```python
from build123d import *

# Parameters (mm, degrees)
SKETCH_W     = 130
SKETCH_H     = 110
PAD_DEPTH    = 1.6
SKETCH001_R  = 1.6
POCKET_DEPTH = 5


with BuildPart() as part:
    # Sketch → Pad (new body)
    with BuildSketch(Plane.XY):
        with Locations((65, 55)):
            Rectangle(SKETCH_W, SKETCH_H)
    extrude(amount=PAD_DEPTH)

    # Sketch001 → Pocket (cut)
    with BuildSketch(Plane.XY):
        with Locations((20, 20)):
            Circle(SKETCH001_R)
        with Locations((110, 89)):
            Circle(SKETCH001_R)
        with Locations((20, 90)):
            Circle(SKETCH001_R)
        with Locations((110, 20)):
            Circle(SKETCH001_R)
    extrude(amount=POCKET_DEPTH, mode=Mode.SUBTRACT)


solid = part.part
```
The listing builds one solid part. Answer for the finished solid, in the listing's coordinates (mm). Coordinates: 2 decimals unless noted, no trailing zeros. Write each loop counter-clockwise with the first axis right and the second up, starting at its lowest first coordinate (ties: lowest second). Pieces come first, ordered by that corner, then holes. Notation, with made-up numbers: (-37, 59) - (11, 59) arc R34 ccw to (11, 96) - close; hole circle Ø2 at (15, 15). An arc over 180 degrees is marked (long way). Return JSON: item names as keys, results as strings. Group by question number.
1. Determine the mould class of faces 1 (the cylindrical face through (19.792, 91.586, 0.789)), 2 (the flat face through (64, 56, 0)) for opening direction X: released by +X, released by -X, zero draft, split by the parting line, or undercut.
2. A cutting plane is placed at B-B, the plane x = 20. Determine the outline of the cut face in (y, z), plus the area to 3 significant figures.
3. Given pin 1 (1.9 mm diameter, centred on x = 20, y = 90, fed in from -Z), flat-ended and moving along its own axis, determine where the tip first touches the part or whether it passes through.
4. A cutting plane is placed at A-A, the plane y = 20. Determine the outline of the cut face in (x, z), plus the area to 3 significant figures.
5. Straight lines are drawn through the part: L1, parallel to X at y = 20, z = 1.2; L2, parallel to Y at x = 20, z = 0.4; L3, parallel to Y at x = 110, z = 0.6. For each, find the intervals that lie inside material, in ascending order.
Ans:
{
 "1": {"face 1": "undercut", "face 2": "zero draft"},
 "2": {"outline": "(0, 0) - (18.4, 0) - (18.4, 1.6) - (0, 1.6) - close; (21.6, 0) - (88.4, 0) - (88.4, 1.6) - (21.6, 1.6) - close; (91.6, 0) - (110, 0) - (110, 1.6) - (91.6, 1.6) - close", "area": "166 mm²"},
 "3": {"pin 1": "through"},
 "4": {"outline": "(0, 0) - (18.4, 0) - (18.4, 1.6) - (0, 1.6) - close; (21.6, 0) - (108.4, 0) - (108.4, 1.6) - (21.6, 1.6) - close; (111.6, 0) - (130, 0) - (130, 1.6) - (111.6, 1.6) - close", "area": "198 mm²"},
 "5": {"L1": "0 to 18.4, 21.6 to 108.4, 111.6 to 130", "L2": "0 to 18.4, 21.6 to 88.4, 91.6 to 110", "L3": "0 to 18.4, 21.6 to 87.4, 90.6 to 110"}
}
